The listing builds one solid part. Answer for the finished solid, in the listing's coordinates (mm). Give positions to 0.01 mm unless a question says otherwise; leave off trailing zeros. Loops run counter-clockwise (first coordinate to the right, second up) from the corner with the lowest first, then second, coordinate; pieces in that order, holes last. Notation, with made-up numbers: M 65.5,47 L 112.5,47 A23 cw 112.5,55 Z; hole C 2,-14.75 d11. An arc over 180 degrees is marked long. Use one line per item in the form item = value. Start each with the question number.
1. The part is cut by section A-A (x = 0). Write down the section's boundary in (y, z), and give its area (3 significant figures).
2. Straight lines are drawn through the part: line 1 (Z direction, x = 0, y = 6); line 2 (Z direction, x = 2.75, y = 6.25); line 3 (Z direction, x = 2, y = 4.5). For each, find the intervals that lie inside material, in ascending order. Write a range as from..to.
3. The part is cut by section D-D (x = 6.75). Write down the section's boundary in (y, z), and give its area (3 significant figures).
4. The mould has two halves that part along Z. Classify faces 1 (the face through (9.436, 3.15, -0.066)), 2 (the face through (1.438, 3.15, -10.955)), 3 (the face through (-5, 6.39, -2)): released by +Z, released by -Z, zero draft, split by the parting line, or undercut.
5. Each of these flat-tipped pins is pushed along its axis until it touches: pin 1 Ø2 at (y, z) = (1, -3) entering from +X; pin 2 Ø2.5 at (x, z) = (0, 7.94) entering from -Y; pin 3 Ø1 at (x, y) = (-2.5, 4.5) entering from +Z; pin 4 Ø1.5 at (x, y) = (-4.5, 2.5) entering from -Z. Where does it stop, or does it pass through?
6. The part is cut by section B-B (z = 0). Write down the section's boundary in (x, y).
7. The part is cut by section C-C (z = 9). Write down the section's boundary in (x, y).
Autodesk Inventor part; units mm, degrees
ref_plane "YZ Plane" through (0, 0, 0) normal (1, 0, 0) x (0, 1, 0)
ref_plane "XZ Plane" through (0, 0, 0) normal (0, 1, 0) x (-1, 0, 0)
ref_plane "XY Plane" through (0, 0, 0) normal (0, 0, 1) x (1, 0, 0)
sketch "Sketch1" plane through (0, 0, 0) normal (0, 1, 0) x (-1, 0, 0)
  circle A0 centre (0, 0) radius 11.049
  circle A1 centre (7.9375, 0) radius 1.5
  circle A2 centre (0, 7.9375) radius 1.5
  circle A3 centre (-7.9375, 0) radius 1.5
  circle A4 centre (0, -7.9375) radius 1.5
  circle A5 centre (0, 0) radius 4.7625
  dimension "d0" = 22.098
  dimension "d1" = 3
  dimension "d2" = 7.9375
  dimension "d5" = 360
  dimension "d7" = 9.525
extrude "Extrusion1" add sketch "Sketch1" along normal blind 6.39
equation "\"d8\" = WoodThickness"
properties part number "CouplingExtender" material "MDF Medium Density Fiberboard"
Derived:
q1.outline = M 0,-11.05 L 6.39,-11.05 L 6.39,-9.44 L 0,-9.44 Z; M 0,-6.44 L 6.39,-6.44 L 6.39,-4.76 L 0,-4.76 Z; M 0,4.76 L 6.39,4.76 L 6.39,6.44 L 0,6.44 Z; M 0,9.44 L 6.39,9.44 L 6.39,11.05 L 0,11.05 Z
q1.area = 42.0 mm2
q2.line_1 = -11.05..-9.44, -6.44..-4.76, 4.76..6.44, 9.44..11.05
q2.line_2 = -10.7..-3.89, 3.89..10.7
q2.line_3 = -10.87..-4.32, 4.32..10.87
q3.outline = M 0,-8.75 L 6.39,-8.75 L 6.39,-0.92 L 0,-0.92 Z; M 0,0.92 L 6.39,0.92 L 6.39,8.75 L 0,8.75 Z
q3.area = 100 mm2
q4.face_1 = undercut
q4.face_2 = split by the parting line
q4.face_3 = zero draft
q5.pin_1 = 10.87
q5.pin_2 = through
q5.pin_3 = 10.87
q5.pin_4 = -10.39
q6.outline = M -11.05,0 L -9.44,0 L -9.44,6.39 L -11.05,6.39 Z; M -6.44,0 L -4.76,0 L -4.76,6.39 L -6.44,6.39 Z; M 4.76,0 L 6.44,0 L 6.44,6.39 L 4.76,6.39 Z; M 9.44,0 L 11.05,0 L 11.05,6.39 L 9.44,6.39 Z
q7.outline = M -6.41,0 L -1.06,0 L -1.06,6.39 L -6.41,6.39 Z; M 1.06,0 L 6.41,0 L 6.41,6.39 L 1.06,6.39 Z
